Source: CAD feature listing. Evaluate the final solid. Frame: model axes, mm. Face numbers are marked on the shaded views. A direction names the side the tool comes from. Round coordinates to 2 decimals unless told otherwise and drop trailing zeros. Write each loop counter-clockwise with the first axis right and the second up, starting at its lowest first coordinate (ties: lowest second). Pieces come first, ordered by that corner, then holes. Notation, with made-up numbers: M 46,-29 L 51,-29 A20 cw 51,-22 Z; hole C 1.5,85.25 d6. An arc over 180 degrees is marked long. Answer in a Markdown table with one row per item.
from build123d import *

# Parameters (mm, degrees)
F0_W           = 8
F0_H           = 53.5
F1_DEPTH       = 4
F2_W           = 8
F2_H           = 52
F2_H_2         = 4
F3_DEPTH       = 4
F5_DEPTH       = 8
F7_DEPTH       = 8
F9_W           = 8
F9_H           = 4
F10_DEPTH      = 20
F11_W          = 4
F11_H          = 8
F12_DEPTH      = 15
F12_DEPTH_BACK = 23


with BuildPart() as f1:
    # F0 (on Front) → F1 (new body)
    with BuildSketch(Plane.XZ):
        with Locations((4, 26.75)):
            Rectangle(F0_W, F0_H)
    extrude(amount=F1_DEPTH)

    # F2 (on face) → F3 (join)
    with BuildSketch(Plane.XY.offset(53.5)):
        with Locations((4, 26)):
            Rectangle(F2_W, F2_H)
        with Locations((4, -2)):
            Rectangle(F2_W, F2_H_2)
    extrude(amount=F3_DEPTH)

    # F4 (on face) → F5 (join)
    with BuildSketch(Plane.YZ.offset(8)):
        Polygon((52, 50), (52, 53.5), (50, 53.5), (50, 52), (47, 52), (47, 50), (50, 50), align=None)
    extrude(amount=-F5_DEPTH)


with BuildPart() as f7:
    # F6 (on face) → F7 (new body)
    with BuildSketch(Plane.YZ.offset(8)):
        Polygon((0, 2), (0, 0), (3.5, 0), (3.5, 2), (3.5, 3.5), (1.5, 3.5), (1.5, 2), align=None)
    extrude(amount=-F7_DEPTH)


with BuildPart() as f1_1:
    add(f1.part)

    # F8: union F7
    add(f7.part)

    # F9 (on face) → F10 (join)
    with BuildSketch(Plane.XZ.offset(4)):
        with Locations((4, 55.5)):
            Rectangle(F9_W, F9_H)
    extrude(amount=F10_DEPTH)

    # F11 (on face) → F12 (join, two sides)
    with BuildSketch(Plane.YZ.offset(8)) as f12_sk:
        with Locations((-2, 49.5)):
            Rectangle(F11_W, F11_H)
        with Locations((-2, 6)):
            Rectangle(F11_W, F11_H)
    extrude(amount=F12_DEPTH)
    extrude(f12_sk.sketch, amount=-F12_DEPTH_BACK)


solid = f1_1.part
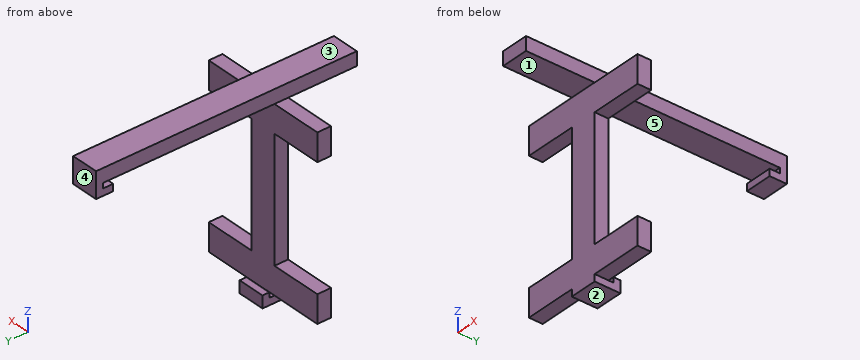
Q1. Access query for the marked faces 1 and 2. Directions: +Z, -Z, +X, -X, +Y, -Y. A direction counts if a zero-diameter tool reaches every point of the face in a straight line with its end or side. Return the directions, or none.
Solutions:
| item | result |
|---|---|
| face 1 | -Z, +X, -X, -Y |
| face 2 | -Z, +X, -X, +Y, -Y |
Q2. Pull-direction query (Y, two-part tool) for the marked faces 3, 4 and 5; classes: pulls with the +Y half, pulls with the -Y half, needs draft (parallel to the pull), parting line crosses it, or undercut.
Solutions:
| item | result |
|---|---|
| face 3 | needs draft |
| face 4 | pulls with the +Y half |
| face 5 | undercut |
Q3. Section C-C (z = 40.5). Return loops of the section in (x, y), and give its area (3 significant figures).
Solutions:
| item | result |
|---|---|
| outline | M 0,-4 L 8,-4 L 8,0 L 0,0 Z |
| area | 32.0 mm2 |
Q4. Contact query for flat-ended pins moving along their axis: pin 1 Ø4 at (x, z) = (3, 24.5) entering from -Y; pin 2 Ø4 at (x, y) = (2.5, -10) entering from -Z; pin 3 Ø1.2 at (y, z) = (-2.5, 32.5) entering from -X. Output: stop coordinate, or through.
Solutions:
| item | result |
|---|---|
| pin 1 | stops at y = -4 |
| pin 2 | stops at z = 53.5 |
| pin 3 | stops at x = 0 |
Q5. Section B-B (y = 2.5). Return loops of the section in (x, z).
Solutions:
| item | result |
|---|---|
| outline | M 0,0 L 8,0 L 8,3.5 L 0,3.5 Z; M 0,53.5 L 8,53.5 L 8,57.5 L 0,57.5 Z |
Q6. Material intervals for probe 1 along Z at (x, y) = (9.5, -2); probe 2 along Y at (x, z) = (16, 52.5); probe 3 along Y at (x, z) = (3, 51), sorted ascending.
Solutions:
| item | result |
|---|---|
| probe 1 | z = 2 to 10, 45.5 to 53.5 |
| probe 2 | y = -4 to 0 |
| probe 3 | y = -4 to 0, 47 to 52 |
Q7. Section A-A (x = -4). Return loops of the section in (y, z).
Solutions:
| item | result |
|---|---|
| outline | M -4,2 L 0,2 L 0,10 L -4,10 Z; M -4,45.5 L 0,45.5 L 0,53.5 L -4,53.5 Z |
Q8. Section D-D (y = 40.5). Return loops of the section in (x, z).
Solutions:
| item | result |
|---|---|
| outline | M 0,53.5 L 8,53.5 L 8,57.5 L 0,57.5 Z |
